```python
from build123d import *

# Parameters (mm, degrees)
SKETCH2_W           = 285
SKETCH2_H           = 258
BOSS_EXTRUDE1_DEPTH = 365
SKETCH3_W           = 275
SKETCH3_H           = 75
CUT_EXTRUDE1_DEPTH  = 35
SKETCH5_W           = 80
SKETCH5_H           = 100
CUT_EXTRUDE2_DEPTH  = 81
SKETCH4_R           = 31.75
CUT_EXTRUDE4_DEPTH  = 276
SKETCH6_W           = 275
SKETCH6_H           = 85
SKETCH6_H_2         = 90
CUT_EXTRUDE6_DEPTH  = 80
SKETCH8_W           = 275
SKETCH8_H           = 163
CUT_EXTRUDE10_DEPTH = 100
SKETCH16_W          = 285
SKETCH16_H          = 255
CUT_EXTRUDE11_DEPTH = 5
SKETCH17_W          = 255
SKETCH17_H          = 230
CUT_EXTRUDE12_DEPTH = 165
SKETCH18_W          = 255
SKETCH18_H          = 10
BOSS_EXTRUDE2_DEPTH = 35
SKETCH19_W          = 20
SKETCH19_H          = 25
BOSS_EXTRUDE3_DEPTH = 35
SKETCH20_W          = 20
SKETCH20_H          = 25
BOSS_EXTRUDE4_DEPTH = 35


with BuildPart() as part:
    # Sketch2 → Boss-Extrude1 (new body)
    with BuildSketch(Plane.XY):
        with Locations((9.388446215, -14.647410359)):
            Rectangle(SKETCH2_W, SKETCH2_H)
    extrude(amount=BOSS_EXTRUDE1_DEPTH)

    # Sketch3 → Cut-Extrude1 (cut)
    with BuildSketch(Plane.XY.offset(365)):
        with Locations((9.388446215, 71.852589641)):
            Rectangle(SKETCH3_W, SKETCH3_H)
    extrude(amount=-CUT_EXTRUDE1_DEPTH, mode=Mode.SUBTRACT)

    # Sketch5 → Cut-Extrude2 (cut)
    with BuildSketch(Plane(origin=(0, 114.352589641, 0), x_dir=(1, 0, 0), z_dir=(0, 1, 0))):
        with Locations((-79.111553785, -60)):
            Rectangle(SKETCH5_W, SKETCH5_H)
        with Locations((8.888446215, -60)):
            Rectangle(SKETCH5_W, SKETCH5_H)
        with Locations((97.888446215, -60)):
            Rectangle(SKETCH5_W, SKETCH5_H)
    extrude(amount=-CUT_EXTRUDE2_DEPTH, mode=Mode.SUBTRACT)

    # Sketch4 → Cut-Extrude4 (cut)
    with BuildSketch(Plane.XY.offset(330)):
        with Locations((-77.411553785, 71.852589641)):
            Circle(SKETCH4_R)
        with Locations((9.388446215, 71.852589641)):
            Circle(SKETCH4_R)
        with Locations((96.188446215, 71.852589641)):
            Circle(SKETCH4_R)
    extrude(amount=-CUT_EXTRUDE4_DEPTH, mode=Mode.SUBTRACT)

    # Sketch6 → Cut-Extrude6 (cut)
    with BuildSketch(Plane(origin=(0, 114.352589641, 0), x_dir=(1, 0, 0), z_dir=(0, 1, 0))):
        with Locations((9.388446215, -187.5)):
            Rectangle(SKETCH6_W, SKETCH6_H)
        with Locations((9.388446215, -280)):
            Rectangle(SKETCH6_W, SKETCH6_H_2)
    extrude(amount=-CUT_EXTRUDE6_DEPTH, mode=Mode.SUBTRACT)

    # Sketch8 → Cut-Extrude10 (cut)
    with BuildSketch(Plane.XY.offset(365)):
        with Locations((9.388446215, -57.147410359)):
            Rectangle(SKETCH8_W, SKETCH8_H)
    extrude(amount=-CUT_EXTRUDE10_DEPTH, mode=Mode.SUBTRACT)

    # Sketch16 → Cut-Extrude11 (cut)
    with BuildSketch(Plane.XZ.offset(143.647410359)):
        with Locations((9.388446215, 132.5)):
            Rectangle(SKETCH16_W, SKETCH16_H)
    extrude(amount=-CUT_EXTRUDE11_DEPTH, mode=Mode.SUBTRACT)

    # Sketch17 → Cut-Extrude12 (cut)
    with BuildSketch(Plane.XZ.offset(138.647410359)):
        with Locations((9.388446215, 130)):
            Rectangle(SKETCH17_W, SKETCH17_H)
    extrude(amount=-CUT_EXTRUDE12_DEPTH, mode=Mode.SUBTRACT)

    # Sketch18 → Boss-Extrude2 (add)
    with BuildSketch(Plane.XZ.offset(-26.352589641)):
        with Locations((9.388446215, 145)):
            Rectangle(SKETCH18_W, SKETCH18_H)
    extrude(amount=BOSS_EXTRUDE2_DEPTH)

    # Sketch19 → Boss-Extrude3 (add, symmetric)
    with BuildSketch(Plane.XZ.offset(-26.352589641)):
        with Locations((9.388446215, 127.5)):
            Rectangle(SKETCH19_W, SKETCH19_H)
    extrude(amount=BOSS_EXTRUDE3_DEPTH, both=True)

    # Sketch20 → Boss-Extrude4 (add, symmetric)
    with BuildSketch(Plane.XZ.offset(-26.352589641)):
        with Locations((-78.111553785, 127.5)):
            Rectangle(SKETCH20_W, SKETCH20_H)
        with Locations((96.888446215, 127.5)):
            Rectangle(SKETCH20_W, SKETCH20_H)
    extrude(amount=BOSS_EXTRUDE4_DEPTH, both=True)


solid = part.part
```
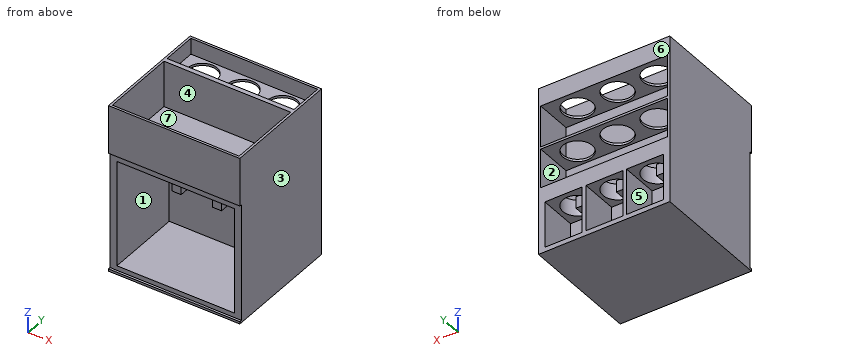
Model file for the job. Use its own axes, mm. Face numbers are marked on the shaded views. A direction names the side the tool comes from. Give positions to 0.01 mm unless a question says otherwise; leave off trailing zeros. Write each loop counter-clockwise with the first axis right and the second up, starting at its lowest first coordinate (ties: lowest second). Pieces come first, ordered by that corner, then holes. Notation, with made-up numbers: (-20.75, 62.5) -> (24.25, 62.5) arc R15 cw to (24.25, 67.5) -> close; hole circle Ø7 at (27.5, 71). An arc over 180 degrees is marked (long way). Use CSV: the item, a comma, the result in double quotes. Start each with the question number.
1) Pin check, flat tips, straight feed: P1, Ø17.5, axis at x = 19, y = 0.5, coming from the +Z side; P2, Ø8, axis at x = -20.5, z = 116.5, coming from the -Y side; P3, Ø16, axis at x = -82, y = 45.5, coming from the +Z side. Stop position of each tip, or through.
2) Cut at C-C on z = 299. List the corners of the cut face in (x, y), plus the area to 4 significant figures.
3) Cut at A-A on y = 17.5. List the corners of the cut face in (x, z), plus the area to 3 significant figures.
4) Cut at B-B on y = -23. List the corners of the cut face in (x, z).
5) Tool access for the marked faces 1, 2, 3 and 4: list every direction of +Z, -Z, +X, -X, +Y, -Y with a clear straight run to the whole face (end or side of a thin tool).
6) Cut at D-D on z = 83.5. List the corners of the cut face in (x, y), plus the area to 3 significant figures.
7) Two-plate mould, pull along Z, no slides. Class the marked faces 5, 6 and 7: released by +Z, released by -Z, zero draft, split by the parting line, or undercut.
8) Drill centre lines: L1, parallel to X at y = 56, z = 81.5; L2, parallel to Z at x = 46, y = -37; L3, parallel to Z at x = -16, y = 8. Where is each one in solid material? Low to high.
Final values:
1,P1,"stops at z = 265"
1,P2,"stops at y = 26.35"
1,P3,"stops at z = 330"
2,outline,"(-133.11, -143.65) -> (151.89, -143.65) -> (151.89, 114.35) -> (146.89, 114.35) -> (146.89, 34.35) -> (-128.11, 34.35) -> (-128.11, 114.35) -> (-133.11, 114.35) -> close; hole (-128.11, -138.65) -> (146.89, -138.65) -> (146.89, 24.35) -> (-128.11, 24.35) -> close"
2,area,"6,705 mm2"
3,outline,"(-133.11, 0) -> (151.89, 0) -> (151.89, 365) -> (146.89, 365) -> (146.89, 265) -> (-128.11, 265) -> (-128.11, 365) -> (-133.11, 365) -> close; hole (-118.11, 15) -> (136.89, 15) -> (136.89, 140) -> (106.89, 140) -> (106.89, 115) -> (86.89, 115) -> (86.89, 140) -> (19.39, 140) -> (19.39, 115) -> (-0.61, 115) -> (-0.61, 140) -> (-68.11, 140) -> (-68.11, 115) -> (-88.11, 115) -> (-88.11, 140) -> (-118.11, 140) -> close; hole (-118.11, 150) -> (136.89, 150) -> (136.89, 245) -> (-118.11, 245) -> close"
3,area,"21,900 mm2"
4,outline,"(-133.11, 0) -> (151.89, 0) -> (151.89, 365) -> (146.89, 365) -> (146.89, 265) -> (-128.11, 265) -> (-128.11, 365) -> (-133.11, 365) -> close; hole (-118.11, 15) -> (136.89, 15) -> (136.89, 245) -> (-118.11, 245) -> close"
5,face 1,"-Y"
5,face 2,"+Y"
5,face 3,"+Z, -Z, +X, +Y, -Y"
5,face 4,"+Z"
6,outline,"(-133.11, -138.65) -> (-118.11, -138.65) -> (-118.11, 26.35) -> (136.89, 26.35) -> (136.89, -138.65) -> (151.89, -138.65) -> (151.89, 114.35) -> (137.89, 114.35) -> (137.89, 33.35) -> (57.89, 33.35) -> (57.89, 114.35) -> (48.89, 114.35) -> (48.89, 33.35) -> (-31.11, 33.35) -> (-31.11, 114.35) -> (-39.11, 114.35) -> (-39.11, 33.35) -> (-119.11, 33.35) -> (-119.11, 114.35) -> (-133.11, 114.35) -> close"
6,area,"10,600 mm2"
7,face 5,"undercut"
7,face 6,"zero draft"
7,face 7,"released by +Z"
8,L1,"x = -133.11 to -119.11, -39.11 to -31.11, 48.89 to 57.89, 137.89 to 151.89"
8,L2,"z = 0 to 15, 245 to 265"
8,L3,"z = 0 to 15, 140 to 150, 245 to 265"
